Verification items for this drawing (mm, ordinates from the low corner). A direction names the side the tool comes from. Round coordinates to 2 decimals unless told otherwise and drop trailing zeros. Order: outer loops, then holes, each group sorted by start corner. A loop starts at its lowest first (then second) coordinate and runs counter-clockwise, first axis right, second up. Notation, with made-up numbers: M 78,-15 L 128,-15 A14 ccw 128,0 Z; hole C 43,40 d1. An arc over 180 degrees is marked long. One line per item, written item: value. Start each with the question number.
(1) Cross-section at C-C, the plane z = 5. Enter the section's corners in (x, y).
(2) Cross-section at A-A, the plane x = 13. Enter the section's corners in (y, z) (3 decimals).
(3) Thickness scan on L1, parallel to Z at x = 22.5, y = 2.6 (3 decimals); L2, parallel to Z at x = 17.75, y = 3.8 (3 decimals); L3, parallel to X at y = 2.9, z = 7. Record the ranges inside material, lowest first.
(4) Release check for a two-part mould opening along Z. For the marked faces 6, 7 and 8 record: released by +Z, released by -Z, zero draft, split by the parting line, or undercut.
(5) Access from +Z, -Z, +X, -X, +Y, -Y to the whole of each face (thin tool, end or side, straight path). Record for the marked faces 1, 2, 3, 4 and 5.
(6) Depth check by flat-ended pin: pin 1 Ø1 at (y, z) = (3, 11.5) entering from -X; pin 2 Ø0.5 at (x, y) = (23, 1.5) entering from +Z. Enter the tip coordinate at first touch or a pass-through.
(7) Cross-section at B-B, the plane y = 3.1. Enter the section's corners in (x, z) (1 decimal).
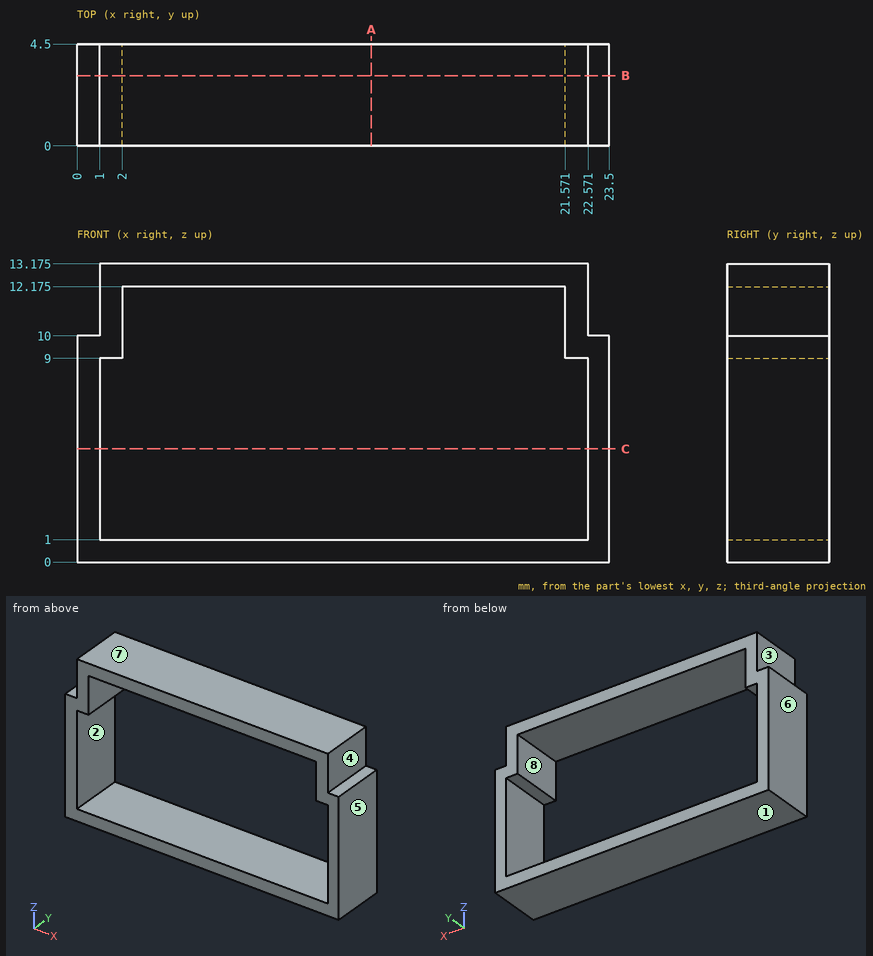
Values found:
1. outline: M 0,0 L 1,0 L 1,4.5 L 0,4.5 Z; M 22.57,0 L 23.5,0 L 23.5,4.5 L 22.57,4.5 Z
2. outline: M 0,0 L 4.5,0 L 4.5,1 L 0,1 Z; M 0,12.175 L 4.5,12.175 L 4.5,13.175 L 0,13.175 Z
3. L1: 0 to 1, 9 to 13.175
3. L2: 0 to 1, 12.175 to 13.175
3. L3: 0 to 1, 22.57 to 23.5
4. face 6: zero draft
4. face 7: released by +Z
4. face 8: undercut
5. face 1: -Z, +X, -X, +Y, -Y
5. face 2: +Y, -Y
5. face 3: +Z, -X, +Y, -Y
5. face 4: +Z, +X, +Y, -Y
5. face 5: +Z, -Z, +X, +Y, -Y
6. pin 1: x = 1
6. pin 2: z = 10
7. outline: M 0,0 L 23.5,0 L 23.5,10 L 22.6,10 L 22.6,13.2 L 1,13.2 L 1,10 L 0,10 Z; hole M 1,1 L 22.6,1 L 22.6,9 L 21.6,9 L 21.6,12.2 L 2,12.2 L 2,9 L 1,9 Z
